from build123d import *

# Parameters (mm, degrees)
SKETCH1_W           = 65.5
SKETCH1_H           = 50
SKETCH1_R           = 4
SKETCH1_R_2         = 1
BOSS_EXTRUDE1_DEPTH = 5
SKETCH3_W           = 5
SKETCH3_H           = 50
BOSS_EXTRUDE2_DEPTH = 85
SKETCH4_R           = 1.025
SKETCH4_W           = 24.4
SKETCH4_H           = 45
CUT_EXTRUDE1_DEPTH  = 66.5


with BuildPart() as part:
    # Sketch1 → Boss-Extrude1 (new body)
    with BuildSketch(Plane(origin=(0, 0, 0), x_dir=(1, 0, 0), z_dir=(0, 1, 0))):
        with Locations((32.75, 25)):
            Rectangle(SKETCH1_W, SKETCH1_H)
        with Locations((49.5, 25)):
            Circle(SKETCH1_R, mode=Mode.SUBTRACT)
        with Locations((49.5, 33)):
            Circle(SKETCH1_R_2, mode=Mode.SUBTRACT)
        with Locations((55.156854249, 30.656854249)):
            Circle(SKETCH1_R_2, mode=Mode.SUBTRACT)
        with Locations((57.5, 25)):
            Circle(SKETCH1_R_2, mode=Mode.SUBTRACT)
        with Locations((55.156854249, 19.343145751)):
            Circle(SKETCH1_R_2, mode=Mode.SUBTRACT)
        with Locations((49.5, 17)):
            Circle(SKETCH1_R_2, mode=Mode.SUBTRACT)
        with Locations((43.843145751, 19.343145751)):
            Circle(SKETCH1_R_2, mode=Mode.SUBTRACT)
        with Locations((41.5, 25)):
            Circle(SKETCH1_R_2, mode=Mode.SUBTRACT)
        with Locations((43.843145751, 30.656854249)):
            Circle(SKETCH1_R_2, mode=Mode.SUBTRACT)
    extrude(amount=BOSS_EXTRUDE1_DEPTH)

    # Sketch3 → Boss-Extrude2 (add)
    with BuildSketch(Plane(origin=(0, 0, 0), x_dir=(1, 0, 0), z_dir=(0, 1, 0))):
        with Locations((2.5, 25)):
            Rectangle(SKETCH3_W, SKETCH3_H)
    extrude(amount=BOSS_EXTRUDE2_DEPTH)

    # Sketch4 → Cut-Extrude1 (cut, through all)
    with BuildSketch(Plane.ZY):
        with Locations((-40, 72.5)):
            Circle(SKETCH4_R)
        with Locations((-10, 72.5)):
            Circle(SKETCH4_R)
        with Locations((-40, 55.5)):
            Circle(SKETCH4_R)
        with Locations((-40, 38.5)):
            Circle(SKETCH4_R)
        with Locations((-10, 55.5)):
            Circle(SKETCH4_R)
        with Locations((-33.5, 32.2)):
            Circle(SKETCH4_R)
        with Locations((-16.5, 32.2)):
            Circle(SKETCH4_R)
        with Locations((-10, 38.5)):
            Circle(SKETCH4_R)
        with Locations((-25, 57.5)):
            Rectangle(SKETCH4_W, SKETCH4_H)
    extrude(amount=-CUT_EXTRUDE1_DEPTH, mode=Mode.SUBTRACT)


solid = part.part
Model file for the job. Use its own axes, mm. A direction names the side the tool comes from. Give positions to 0.01 mm unless a question says otherwise; leave off trailing zeros. Loops run counter-clockwise (first coordinate to the right, second up) from the corner with the lowest first, then second, coordinate; pieces in that order, holes last.
Item 1: Drill centre lines: line 1 along Y through (x, z) = (2.7, -10) (3 decimals); line 2 along X through (y, z) = (2.25, -25); line 3 along Y through (x, z) = (59, -7). Where is each one in solid material? Low to high.
Check values:
line 1: y = 0 to 37.475, 39.525 to 54.475, 56.525 to 71.475, 73.525 to 85
line 2: x = 0 to 40.5, 42.5 to 45.5, 53.5 to 56.5, 58.5 to 65.5
line 3: y = 0 to 5
Item 2: Slice it at D-D (z = -27). Write the cut outline in (x, y), plus the area to 3 significant figures.
Check values:
outline: (0, 0) - (46.04, 0) - (46.04, 5) - (5, 5) - (5, 35) - (0, 35) - close; (0, 80) - (5, 80) - (5, 85) - (0, 85) - close; (52.96, 0) - (65.5, 0) - (65.5, 5) - (52.96, 5) - close
area: 468 mm2
Item 3: Which spindle directions (+Z, -Z, +X, -X, +Y, -Y) get a long thin tool onto all of the face, cutting with end or side? Do faces 3 (the face through (2, 57, -12.8)), 4 (the face through (56.11, 2.46, -30.96)). Say none if no direction does.
Check values:
face 3: +X, -X
face 4: +Y, -Y
Item 4: Drop flat-ended pins along their axis: P1, Ø2.5, axis at x = 55.16, z = -30.66, coming from the +Y side; P2, Ø1.2, axis at y = 55.5, z = -40, coming from the +X side; P3, Ø15, axis at y = 44.5, z = -16.5, coming from the +X side. Give the stop position or say it passes through.
Check values:
P1: stops at y = 5
P2: passes through
P3: stops at x = 5
Item 5: Slice it at A-A (z = -40). Write the cut outline in (x, y) (3 decimals), plus the area to 3 significant figures.
Check values:
outline: (0, 0) - (65.5, 0) - (65.5, 5) - (5, 5) - (5, 37.475) - (0, 37.475) - close; (0, 39.525) - (5, 39.525) - (5, 54.475) - (0, 54.475) - close; (0, 56.525) - (5, 56.525) - (5, 71.475) - (0, 71.475) - close; (0, 73.525) - (5, 73.525) - (5, 85) - (0, 85) - close
area: 697 mm2
Item 6: Mould opens along Z. For faces 1 (the face through (2, 57, -37.2)), 2 (the face through (2, 85, -25)) say: +Z half, -Z half, draft (parallel to the pull), parting line (faces both ways), or undercut.
Check values:
face 1: undercut
face 2: draft
Item 7: Slice it at C-C (y = 49). Write the cut outline in (x, z).
Check values:
outline: (0, -50) - (5, -50) - (5, -37.2) - (0, -37.2) - close; (0, -12.8) - (5, -12.8) - (5, 0) - (0, 0) - close
Item 8: Slice it at B-B (x = 41.5). Write the cut outline in (y, z).
Check values:
outline: (0, -50) - (5, -50) - (5, -26) - (0, -26) - close; (0, -24) - (5, -24) - (5, 0) - (0, 0) - close
